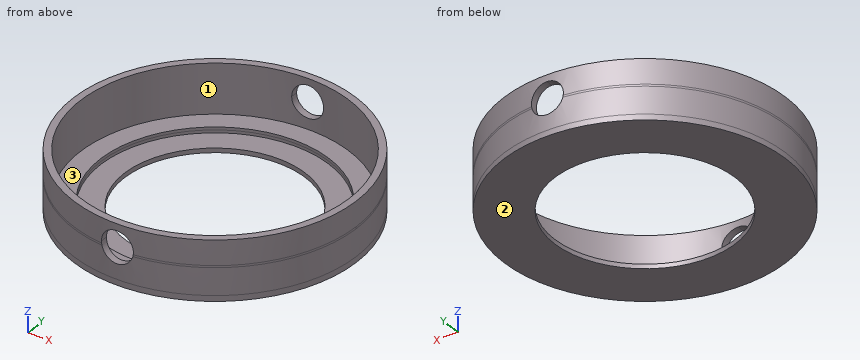
Autodesk Inventor part; units mm, degrees
ref_plane "Work Plane1" through (0, 25, 0) normal (0, 1, 0) x (-1, 0, 0)
ref_plane "YZ Plane" through (0, 0, 0) normal (1, 0, 0) x (0, 1, 0)
ref_plane "XY Plane" through (0, 0, 0) normal (0, 0, 1) x (1, 0, 0)
sketch "Sketch1" plane through (0, 0, 0) normal (0, 0, 1) x (1, 0, 0)
  circle A0 centre (0, 0) radius 25
  dimension "d0" = 50
extrude "Initial Cylinder" add sketch "Sketch1" along normal blind 4.78
sketch "Sketch2" plane through (0, 0, 4.78) normal (0, 0, 1) x (1, 0, 0)
  circle A0 centre (0, 0) radius 16
  dimension "d3" = 32
extrude "Through-hole" cut sketch "Sketch2" against normal blind 548
sketch "Sketch3" plane through (0, 0, 4.78) normal (0, 0, 1) x (1, 0, 0)
  circle A0 centre (0, 0) radius 23.75
  dimension "d6" = 47.5
extrude "snug ring fit" cut sketch "Sketch3" against normal blind 4
sketch "Sketch5" plane through (0, 0, 0) normal (0, 1, 0) x (-1, 0, 0)
  line L0 (25, 4.78) -> (-25, 4.78)
  line L1 (25, 0) -> (-25, 0)
  point P0 (0, 0)
  dimension "d16" = 4.78
sketch "Sketch6" plane through (0, 0, 0.78) normal (0, 0, 1) x (1, 0, 0)
  circle A0 centre (0, 0) radius 20.2
  dimension "d17" = 40.4
extrude "Extrusion5" cut sketch "Sketch6" against normal blind 0.5
sketch "Sketch7" plane through (0, 0, 0) normal (0, 0, -1) x (-1, 0, 0)
  circle A0 centre (0, 0) radius 16
  circle A1 centre (0, 0) radius 25
extrude "Extrusion6" add sketch "Sketch7" along normal blind 1
sketch "Sketch8" plane through (0, 0, 0.28) normal (0, 0, 1) x (1, 0, 0)
  circle A0 centre (0, 0) radius 16
  circle A1 centre (0, 0) radius 20.2
  circle A2 centre (0, 0) radius 17.75
  dimension "d26" = 35.5
extrude "Extrusion7" cut sketch "Sketch8" along normal mid plane 1 contours A0 | A1 | A2
sketch "Sketch9" plane through (0, 0, 4.78) normal (0, 0, 1) x (1, 0, 0)
  circle A0 centre (0, 0) radius 23.75
  circle A1 centre (0, 0) radius 25
extrude "Extrusion8" add sketch "Sketch9" along normal blind 0.35
sketch "Sketch10" plane through (0, 0, 5.13) normal (0, 0, 1) x (1, 0, 0)
  circle A0 centre (0, 0) radius 23.75
  circle A1 centre (0, 0) radius 25
  dimension "d30" = 1.25
extrude "Extrusion9" add sketch "Sketch10" along normal blind 4.38
sketch "Sketch4" plane through (0, 0, 0) normal (0, 1, 0) x (-1, 0, 0)
  line L0 (25, 4.78) -> (-25, 4.78)
  line L1 (0, 4.78) -> (0, 5.78)
  circle A0 centre (0, 5.78) radius 2.825
  point P0 (0, 0)
  dimension "d10" = 5.65
  dimension "d29" = 1
extrude "Extrusion4" [suppressed]
ref_plane "Work Plane1" through (0, 25, 0) normal (0, 1, 0) x (-1, 0, 0)
sketch "Sketch11" plane through (0, 25, 0) normal (0, 1, 0) x (-1, 0, 0)
  line L0 (16, -0.22) -> (-16, -0.22)
  line L1 (25, 9.51) -> (-25, 9.51)
  line L2 (-23.75, 9.51) -> (23.75, 9.51)
  line L3 (0, 9.51) -> (0, 5.51)
  circle A0 centre (0, 5.51) radius 2.825
  point P0 (0, 0)
  dimension "d32" = 9.73
  dimension "d33" = 4
  dimension "d34" = 5.65
extrude "Extrusion10" cut sketch "Sketch11" along normal mid plane 1000
properties part number "Diaphragm_lock"
Work out the finished part from the listing and answer in its coordinate system (mm). Face numbers are marked on the shaded views. Round coordinates to 2 decimals unless told otherwise and drop trailing zeros. Write each loop counter-clockwise with the first axis right and the second up, starting at its lowest first coordinate (ties: lowest second). Pieces come first, ordered by that corner, then holes. Notation, with made-up numbers: (80, 8) -> (118, 8) arc R19 ccw to (118, 37) -> close; hole circle Ø9 at (84, -32.5). An arc over 180 degrees is marked (long way). Write each question's results on one line, items separated by ' | '.
1) The part is cut by section D-D (y = -18.5). Write down the section's boundary in (x, z), and give its area (3 significant figures).
Findings:
outline: (-16.82, -1) -> (16.82, -1) -> (16.82, 9.51) -> (14.89, 9.51) -> (14.89, 0.78) -> (8.11, 0.78) -> (8.11, -0.22) -> (-8.11, -0.22) -> (-8.11, 0.78) -> (-14.89, 0.78) -> (-14.89, 9.51) -> (-16.82, 9.51) -> close | area: 77.2 mm²
2) The part is cut by section B-B (y = -9). Write down the section's boundary in (x, z), and give its area (3 significant figures).
Findings:
outline: (-23.32, -1) -> (-13.23, -1) -> (-13.23, -0.22) -> (-18.08, -0.22) -> (-18.08, 0.78) -> (-21.98, 0.78) -> (-21.98, 9.51) -> (-23.32, 9.51) -> close; (13.23, -1) -> (23.32, -1) -> (23.32, 9.51) -> (21.98, 9.51) -> (21.98, 0.78) -> (18.08, 0.78) -> (18.08, -0.22) -> (13.23, -0.22) -> close | area: 49.7 mm²
3) Flat-ended cylindrical pins translate along their axes: pin 1 (24 mm diameter, centred on x = 0, y = 0, fed in from +Z); pin 2 (20 mm diameter, centred on x = 1.5, y = -9.5, fed in from +Z); pin 3 (5 mm diameter, centred on y = 12.5, z = 6, fed in from -X); pin 4 (5 mm diameter, centred on y = 16, z = 8.5, fed in from -X). Find the tip coordinate at first contact, or state that the pin passes through.
Findings:
pin 1: passes through | pin 2: stops at z = -0.22 | pin 3: stops at x = -22.91 | pin 4: stops at x = -21.04
4) The part is cut by section A-A (x = -15). Write down the section's boundary in (y, z).
Findings:
outline: (-20, -1) -> (-5.57, -1) -> (-5.57, -0.22) -> (-13.53, -0.22) -> (-13.53, 0.78) -> (-18.41, 0.78) -> (-18.41, 9.51) -> (-20, 9.51) -> close; (5.57, -1) -> (20, -1) -> (20, 9.51) -> (18.41, 9.51) -> (18.41, 0.78) -> (13.53, 0.78) -> (13.53, -0.22) -> (5.57, -0.22) -> close
5) The part is cut by section C-C (z = 1.5). Write down the section's boundary in (x, y), and give its area (3 significant figures).
Findings:
outline: circle Ø50 at (0, 0); hole circle Ø47.5 at (0, 0) | area: 191 mm²
6) Consider line 1 along Z through (x, y) = (0, 23.9) (3 decimals); line 2 along Y through (x, z) = (0, -0.1); line 3 along Z through (x, y) = (19.5, 11). Determine where each line is inside the solid, lowest interval first. Write a range as [from, to].
Findings:
line 1: z = [-1, 2.685], [8.335, 9.51] | line 2: y = [-25, -20.2], [20.2, 25] | line 3: z = [-1, 0.78]
7) For a pull along X with two mould halves and no side action, classify the marked faces 1, 2 and 3 as +X half, -X half, draft (parallel to the pull), parting line (faces both ways), or undercut.
Findings:
face 1: undercut | face 2: draft | face 3: undercut
